Design review of the part shown in the three views and the two pictorial views. Dimensions are in mm from the part's minimum x, y and z. Coordinates: 2 decimals unless noted, no trailing zeros. Write each loop counter-clockwise with the first axis right and the second up, starting at its lowest first coordinate (ties: lowest second). Pieces come first, ordered by that corner, then holes. Notation, with made-up numbers: (25, -9) - (49, -9) arc R29 ccw to (49, 25) - close; hole circle Ø6 at (86, -37.5). An arc over 180 degrees is marked (long way). Write each question's results on one line, items separated by ' | '.
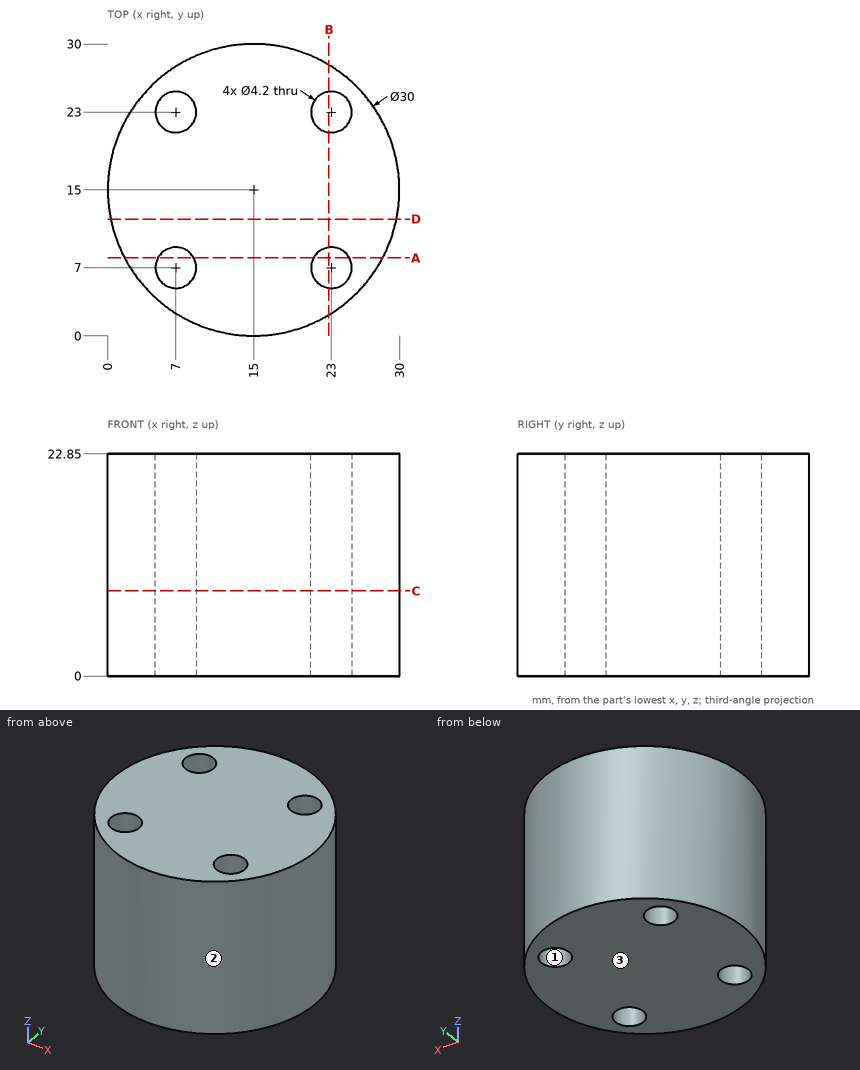
Q1. For pin 1 (1.5 mm diameter, centred on x = 16, y = 21.5, fed in from -Z); pin 2 (12 mm diameter, centred on x = 8, z = 8, fed in from -Y); pin 3 (4 mm diameter, centred on x = 7, y = 23, fed in from +Z); pin 4 (12 mm diameter, centred on x = 21.5, z = 15, fed in from +Y), all flat-tipped, find the tip position at first contact; note any pin that passes through.
Results found:
pin 1: z = 0 | pin 2: y = 0.03 | pin 3: through | pin 4: y = 29.99
Q2. Mouldability with a two-part tool opening along X and no side actions: class the marked faces 1, 2 and 3 as pulls with the +X half, pulls with the -X half, needs draft (parallel to the pull), parting line crosses it, or undercut.
Results found:
face 1: undercut | face 2: parting line crosses it | face 3: needs draft
Q3. Take a section at B-B on x = 22.75. State the section outline as (y, z) points.
Results found:
outline: (2.16, 0) - (4.91, 0) - (4.91, 22.85) - (2.16, 22.85) - close; (9.09, 0) - (20.91, 0) - (20.91, 22.85) - (9.09, 22.85) - close; (25.09, 0) - (27.84, 0) - (27.84, 22.85) - (25.09, 22.85) - close
Q4. Take a section at A-A on y = 8. State the section outline as (x, z) points, plus the area to 3 significant figures.
Results found:
outline: (1.73, 0) - (5.15, 0) - (5.15, 22.85) - (1.73, 22.85) - close; (8.85, 0) - (21.15, 0) - (21.15, 22.85) - (8.85, 22.85) - close; (24.85, 0) - (28.27, 0) - (28.27, 22.85) - (24.85, 22.85) - close | area: 437 mm2
Q5. Take a section at D-D on y = 12. State the section outline as (x, z) points.
Results found:
outline: (0.3, 0) - (29.7, 0) - (29.7, 22.85) - (0.3, 22.85) - close
Q6. Take a section at C-C on z = 8.75. State the section outline as (x, y) points.
Results found:
outline: circle Ø30 at (15, 15); hole circle Ø4.2 at (7, 7); hole circle Ø4.2 at (7, 23); hole circle Ø4.2 at (23, 7); hole circle Ø4.2 at (23, 23)
Q7. Wall thickness on line 1 along Y through (x, z) = (7, 18); line 2 along Y through (x, z) = (21.25, 4.75); line 3 along X through (y, z) = (5.5, 6): over which ranges is each line inside the solid? List them lowest first. Write a range as from..to.
Results found:
line 1: 2.31..4.9, 9.1..20.9, 25.1..27.69 | line 2: 1.36..5.84, 8.16..21.84, 24.16..28.64 | line 3: 3.39..5.53, 8.47..21.53, 24.47..26.61
